from build123d import *

# Parameters (mm, degrees)
SKETCH005_W  = 13.9
SKETCH005_H  = 13.9
PAD006_DEPTH = 10
SKETCH006_W  = 13.9
SKETCH006_H  = 13.9
PAD007_DEPTH = 1.3
PAD008_DEPTH = 2.7
PAD009_DEPTH = 10
SKETCH009_W  = 13.9
SKETCH009_H  = 13.9
PAD011_DEPTH = 10
SKETCH010_W  = 13.9
SKETCH010_H  = 13.9
PAD012_DEPTH = 1.3
PAD013_DEPTH = 2.7
PAD014_DEPTH = 10
SKETCH001_W  = 13.9
SKETCH001_H  = 13.9
PAD001_DEPTH = 10
SKETCH002_W  = 13.9
SKETCH002_H  = 13.9
PAD002_DEPTH = 1.3
PAD003_DEPTH = 2.7
PAD004_DEPTH = 10
PAD015_DEPTH = 9.5


with BuildPart() as subtractormiddle:
    with BuildSketch(Plane(origin=(0, 0.025, 2), x_dir=(0, -1, 0), z_dir=(0, 0, 1))):
        Rectangle(SKETCH005_W, SKETCH005_H)
    extrude(amount=PAD006_DEPTH)

    # Sketch006 (on Face5 of Pad006) → Pad007 (join)
    with BuildSketch(Plane(origin=(0, 0.025, 2), x_dir=(0, -1, 0), z_dir=(0, 0, -1))):
        Rectangle(SKETCH006_W, SKETCH006_H)
    extrude(amount=PAD007_DEPTH)

    # Sketch007 (on Face9 of Pad007) → Pad008 (join)
    with BuildSketch(Plane(origin=(0, 0.025, 0.7), x_dir=(0, -1, 0), z_dir=(0, 0, -1))):
        Polygon((-6.95, 6.95), (-6.95, 2.5), (-7.45, 2.5), (-7.45, -2.5), (-6.95, -2.5), (-6.95, -6.95), (6.95, -6.95), (6.95, -2.5), (7.45, -2.5), (7.45, 2.5), (6.95, 2.5), (6.95, 6.95), align=None)
    extrude(amount=PAD008_DEPTH)

    # Sketch007 (on Face9 of Pad007) → Pad009 (join)
    with BuildSketch(Plane(origin=(0, 0.025, 0.7), x_dir=(0, -1, 0), z_dir=(0, 0, -1))):
        Polygon((-6.95, 6.95), (-6.95, 2.5), (-7.45, 2.5), (-7.45, -2.5), (-6.95, -2.5), (-6.95, -6.95), (6.95, -6.95), (6.95, -2.5), (7.45, -2.5), (7.45, 2.5), (6.95, 2.5), (6.95, 6.95), align=None)
    extrude(amount=PAD009_DEPTH)


with BuildPart() as subtractorbottom:
    with BuildSketch(Plane(origin=(0, -21.350023, 4.719246), x_dir=(0, -0.968148, 0.25038), z_dir=(0, 0.25038, 0.968148))):
        Rectangle(SKETCH009_W, SKETCH009_H)
    extrude(amount=PAD011_DEPTH)

    # Sketch010 (on Face5 of Pad011) → Pad012 (join)
    with BuildSketch(Plane(origin=(0, -21.350023, 4.719246), x_dir=(0, -0.968148, 0.25038), z_dir=(0, -0.25038, -0.968148))):
        Rectangle(SKETCH010_W, SKETCH010_H)
    extrude(amount=PAD012_DEPTH)

    # Sketch011 (on Face9 of Pad012) → Pad013 (join)
    with BuildSketch(Plane(origin=(0, -21.675517, 3.460654), x_dir=(0, -0.968148, 0.25038), z_dir=(0, -0.25038, -0.968148))):
        Polygon((-6.95, 6.95), (-6.95, 2.5), (-7.45, 2.5), (-7.45, -2.5), (-6.95, -2.5), (-6.95, -6.95), (6.95, -6.95), (6.95, -2.5), (7.45, -2.5), (7.45, 2.5), (6.95, 2.5), (6.95, 6.95), align=None)
    extrude(amount=PAD013_DEPTH)

    # Sketch011 (on Face9 of Pad012) → Pad014 (join)
    with BuildSketch(Plane(origin=(0, -21.675517, 3.460654), x_dir=(0, -0.968148, 0.25038), z_dir=(0, -0.25038, -0.968148))):
        Polygon((-6.95, 6.95), (-6.95, 2.5), (-7.45, 2.5), (-7.45, -2.5), (-6.95, -2.5), (-6.95, -6.95), (6.95, -6.95), (6.95, -2.5), (7.45, -2.5), (7.45, 2.5), (6.95, 2.5), (6.95, 6.95), align=None)
    extrude(amount=PAD014_DEPTH)


with BuildPart() as refinedsubtractorcompound2:
    with BuildSketch(Plane(origin=(0.025, 21.301615, 4.706727), x_dir=(0, -0.968148, -0.25038), z_dir=(0, -0.25038, 0.968148))):
        Rectangle(SKETCH001_W, SKETCH001_H)
    extrude(amount=PAD001_DEPTH)

    # Sketch002 (on Face5 of Pad001) → Pad002 (join)
    with BuildSketch(Plane(origin=(0.025, 21.301615, 4.706727), x_dir=(0, -0.968148, -0.25038), z_dir=(0, 0.25038, -0.968148))):
        Rectangle(SKETCH002_W, SKETCH002_H)
    extrude(amount=PAD002_DEPTH)

    # Sketch003 (on Face9 of Pad002) → Pad003 (join)
    with BuildSketch(Plane(origin=(0.025, 21.627109, 3.448135), x_dir=(0, -0.968148, -0.25038), z_dir=(0, 0.25038, -0.968148))):
        Polygon((-6.95, 6.95), (-6.95, 2.5), (-7.45, 2.5), (-7.45, -2.5), (-6.95, -2.5), (-6.95, -6.95), (6.95, -6.95), (6.95, -2.5), (7.45, -2.5), (7.45, 2.5), (6.95, 2.5), (6.95, 6.95), align=None)
    extrude(amount=PAD003_DEPTH)

    # Sketch003 (on Face9 of Pad002) → Pad004 (join)
    with BuildSketch(Plane(origin=(0.025, 21.627109, 3.448135), x_dir=(0, -0.968148, -0.25038), z_dir=(0, 0.25038, -0.968148))):
        Polygon((-6.95, 6.95), (-6.95, 2.5), (-7.45, 2.5), (-7.45, -2.5), (-6.95, -2.5), (-6.95, -6.95), (6.95, -6.95), (6.95, -2.5), (7.45, -2.5), (7.45, 2.5), (6.95, 2.5), (6.95, 6.95), align=None)
    extrude(amount=PAD004_DEPTH)

    # Compound: union SubtractorMiddle, SubtractorBottom
    add(subtractormiddle.part)
    add(subtractorbottom.part)


with BuildPart() as obj1:
    # Sketch012 → Pad015 (new body, symmetric)
    with BuildSketch(Plane.YZ):
        with BuildLine():
            Line((-9.525, 2), (9.525, 2))
            Line((9.525, 2), (12.104213, 2.328117))
            Line((12.104213, 2.328117), (30.547425, 7.097856))
            Line((30.547425, 7.097856), (33.126638, 7.425974))
            ThreePointArc((34.889388, 7.537649), (34.006246, 7.509702), (33.126638, 7.425974))
            Line((60.889388, 7.537649), (34.889388, 7.537649))
            Line((60.889388, 3.569629), (60.889388, 7.537649))
            Line((34.889388, 3.569629), (60.889388, 3.569629))
            ThreePointArc((34.889388, 3.569629), (34.257128, 3.549621), (33.627398, 3.489678))
            Line((31.548945, 3.225266), (33.627398, 3.489678))
            Line((13.105733, -1.544473), (31.548945, 3.225266))
            Line((9.525, -2), (13.105733, -1.544473))
            Line((-9.525, -2), (9.525, -2))
            Line((-13.105733, -1.544473), (-9.525, -2))
            Line((-31.548945, 3.225266), (-13.105733, -1.544473))
            Line((-31.548945, 3.225266), (-33.627398, 3.489678))
            ThreePointArc((-33.627398, 3.489678), (-35.573549, 3.35359), (-37.31948, 2.483102))
            Line((-52.342581, -9.149027), (-37.31948, 2.483102))
            Line((-54.771872, -6.011555), (-52.342581, -9.149027))
            Line((-39.74877, 5.620573), (-54.771872, -6.011555))
            ThreePointArc((-33.126638, 7.425974), (-36.617262, 7.181886), (-39.74877, 5.620573))
            Line((-30.547425, 7.097856), (-33.126638, 7.425974))
            Line((-12.104213, 2.328117), (-30.547425, 7.097856))
            Line((-9.525, 2), (-12.104213, 2.328117))
        make_face()
    extrude(amount=PAD015_DEPTH, both=True)

    # Cut002: cut RefinedSubtractorCompound2
    add(refinedsubtractorcompound2.part, mode=Mode.SUBTRACT)


solid = obj1.part
Design review of the part built by this model. Coordinates are the model's own, in mm. A direction names the side the tool comes from. Give positions to 0.01 mm unless a question says otherwise; leave off trailing zeros. Write each loop counter-clockwise with the first axis right and the second up, starting at its lowest first coordinate (ties: lowest second). Pieces come first, ordered by that corner, then holes. Notation, with made-up numbers: M 69,13.25 L 117,13.25 A23 cw 117,24.25 Z; hole C 39.5,29.25 d5. An arc over 180 degrees is marked long. Return JSON: item names as keys, results as strings. Group by question number.
Item 1: The part is to be moulded in two halves that separate along Y. For faces 4 (the flat face through (0.133, -47.155, -0.114)), 5 (the flat face through (0.06, 14.75, 0.29)), 6 (the flat face through (6.95, 0, 0)), 7 (the flat face through (0, 48, 7.538)), say which applies: pulls with the +Y half, pulls with the -Y half, needs draft (parallel to the pull), parting line crosses it, or undercut.
Item 2: Take a section at D-D (z = -3.5). Give the boundary of the cut face in (x, y), plus the area to 3 significant figures.
Item 3: Clearance check with flat-ended pins moving along their axes: pin 1 Ø2 at (x, z) = (-6.5, -5) entering from +Y; pin 2 Ø8 at (x, y) = (4.5, 45.5) entering from -Z; pin 3 Ø1.4 at (x, z) = (-0.5, 0) entering from -Y. State where each tip first meets the part, or that it passes through.
Item 4: Tool access review of faces 1 (the flat face through (-6.95, 0, 0)), 2 (the flat face through (-8, 0, -2)), 3 (the flat face through (0.133, -10.797, 2.162)): name each direction out of +Z, -Z, +X, -X, +Y, -Y from which nothing blocks a thin tool from reaching the whole face with its end or side.
Item 5: Wall thickness on line 1 along Y through (x, z) = (4.25, 1.5) (3 decimals); line 2 along X through (y, z) = (19.5, 0.25) (3 decimals); line 3 along Y through (x, z) = (-3.5, 0.5) (3 decimals): over which ranges is each line inside the solid? List them lowest first.
Item 6: Take a section at A-A (y = -18). Give the boundary of the cut face in (x, z).
Item 7: Take a section at B-B (x = -3.75). Count the separate pieces of the cut face and the enclosed holes in it, plus the area to 3 significant figures.
Item 8: Take a section at C-C (y = 38.5). Give the boundary of the cut face in (x, z).
Return value:
{
 "1": {"face 4": "pulls with the -Y half", "face 5": "pulls with the +Y half", "face 6": "undercut", "face 7": "needs draft"},
 "2": {"outline": "M -9.5,-51.53 L 9.5,-51.53 L 9.5,-45.05 L -9.5,-45.05 Z", "area": "123 mm2"},
 "3": {"pin 1": "stops at y = -45.69", "pin 2": "stops at z = 3.57", "pin 3": "stops at y = -47.91"},
 "4": {"face 1": "+Z, -Z", "face 2": "-Z, +X, -X, +Y", "face 3": "+Z, +X, -X"},
 "5": {"line 1": "y = -45.071 to -38.589, -15.004 to -6.925, 6.975 to 14.952", "line 2": "x = -9.5 to -6.925, 6.975 to 9.5", "line 3": "y = -46.362 to -39.881, -15.263 to -6.925, 6.975 to 15.211"},
 "6": {"outline": "M -9.5,-0.28 L -6.95,-0.28 L -6.95,3.85 L -9.5,3.85 Z; M 6.95,-0.28 L 9.5,-0.28 L 9.5,3.85 L 6.95,3.85 Z"},
 "7": {"separate pieces": "4", "enclosed holes": "0", "area": "311 mm2"},
 "8": {"outline": "M -9.5,3.57 L 9.5,3.57 L 9.5,7.54 L -9.5,7.54 Z"}
}
